from build123d import *

# Parameters (mm, degrees)
SKETCH1_W           = 12.7
SKETCH1_H           = 12.7
SKETCH1_R           = 1.905
BOSS_EXTRUDE1_DEPTH = 2.54
SKETCH2_W           = 1.791864934
SKETCH2_H           = 1.49598957
BOSS_EXTRUDE2_DEPTH = 10.16
SKETCH3_R           = 1.375
CUT_EXTRUDE1_DEPTH  = 17.896123524
FILLET1_R           = 1.016


with BuildPart() as part:
    # Sketch1 → Boss-Extrude1 (new body)
    with BuildSketch(Plane(origin=(0, 0, 0), x_dir=(1, 0, 0), z_dir=(0, 1, 0))):
        Rectangle(SKETCH1_W, SKETCH1_H)
        with Locations(Location((-3.175, 3.175, 0), (0, 0, 270))):
            Circle(SKETCH1_R, mode=Mode.SUBTRACT)
        with Locations(Location((3.175, 3.175, 0), (0, 0, 90))):
            Circle(SKETCH1_R, mode=Mode.SUBTRACT)
        with Locations(Location((3.175, -3.175, 0), (0, 0, 270))):
            Circle(SKETCH1_R, mode=Mode.SUBTRACT)
        with Locations(Location((-3.175, -3.175, 0), (0, 0, 90))):
            Circle(SKETCH1_R, mode=Mode.SUBTRACT)
    extrude(amount=BOSS_EXTRUDE1_DEPTH)

    # Sketch2 → Boss-Extrude2 (add)
    with BuildSketch(Plane(origin=(0, 2.54, 0), x_dir=(1, 0, 0), z_dir=(0, 1, 0))):
        Polygon((-1.016, 0.747994785), (-1.016, 2.249760645), (-2.807864934, 0.747994785), align=None)
        with Locations((-1.911932467, 0)):
            Rectangle(SKETCH2_W, SKETCH2_H)
        Polygon((-1.016, -2.249760645), (-1.016, -0.747994785), (-2.807864934, -0.747994785), align=None)
        Polygon((2.807864934, 0.747994785), (1.016, 2.249760645), (1.016, 0.747994785), align=None)
        with Locations((1.911932467, 0)):
            Rectangle(SKETCH2_W, SKETCH2_H)
        Polygon((2.807864934, -0.747994785), (1.016, -0.747994785), (1.016, -2.249760645), align=None)
    extrude(amount=BOSS_EXTRUDE2_DEPTH)

    # Sketch3 → Cut-Extrude1 (cut, through all)
    with BuildSketch(Plane(origin=(2.807864934, 0, 0), x_dir=(0, 0, -1), z_dir=(1, 0, 0))):
        with Locations(Location((0, 6.35, 0), (0, 0, 57.043905398))):
            Circle(SKETCH3_R)
    extrude(amount=-CUT_EXTRUDE1_DEPTH, mode=Mode.SUBTRACT)

    # Fillet1
    fillet1_edges = [part.edges().sort_by_distance(p)[0] for p in [
        (-6.35, 2.54, 0),
        (0, 2.54, 6.35),
        (6.35, 2.54, 0),
        (6.35, 1.27, 6.35),
        (-6.35, 1.27, 6.35),
        (-6.35, 1.27, -6.35),
        (6.35, 1.27, -6.35),
        (0, 2.54, -6.35),
    ]]
    fillet(fillet1_edges, radius=FILLET1_R)


solid = part.part
Read the model definition and answer for the solid it produces. Units are mm, in the model's axes. A direction names the side the tool comes from. Round coordinates to 2 decimals unless told otherwise and drop trailing zeros. Write each loop counter-clockwise with the first axis right and the second up, starting at its lowest first coordinate (ties: lowest second). Pieces come first, ordered by that corner, then holes.
Q1. Find section B-B on z = -0.5. Determine the outline of the cut face in (x, y), and give its area (3 significant figures).
Values:
outline: (-6.35, 0) - (6.35, 0) - (6.35, 1.52) arc R1.02 ccw to (5.33, 2.54) - (2.81, 2.54) - (2.81, 5.07) - (1.02, 5.07) - (1.02, 2.54) - (-1.02, 2.54) - (-1.02, 5.07) - (-2.81, 5.07) - (-2.81, 2.54) - (-5.33, 2.54) arc R1.02 ccw to (-6.35, 1.52) - close; (-2.81, 7.63) - (-1.02, 7.63) - (-1.02, 12.7) - (-2.81, 12.7) - close; (1.02, 7.63) - (2.81, 7.63) - (2.81, 12.7) - (1.02, 12.7) - close
area: 59.0 mm2
Q2. The mould has two halves that part along X. Classify faces 1 (the face through (6, 0.8, -6.1)), 2 (the face through (-3.905, 1.252, -1.415)), 3 (the face through (0, 0, 0)), 4 (the face through (5.064, 1.252, 2.927)): released by +X, released by -X, zero draft, split by the parting line, or undercut.
Values:
face 1: released by +X
face 2: undercut
face 3: zero draft
face 4: undercut
Q3. Straight lines are drawn through the part: line 1 (X direction, y = 2.75, z = 0); line 2 (Z direction, x = -2.5, y = 0.5); line 3 (Y direction, x = -1.25, z = -0.75). For each, find the intervals that lie inside material, in ascending order.
Values:
line 1: x = -2.81 to -1.02, 1.02 to 2.81
line 2: z = -6.35 to -4.96, -1.39 to 1.39, 4.96 to 6.35
line 3: y = 0 to 5.2, 7.5 to 12.7
Q4. Find section C-C on y = 7. Determine the outline of the cut face in (x, z), and give its area (3 significant figures).
Values:
outline: (-2.25, -1.21) - (-1.02, -2.25) - (-1.02, -1.21) - close; (-2.25, 1.21) - (-1.02, 1.21) - (-1.02, 2.25) - close; (1.02, -2.25) - (2.25, -1.21) - (1.02, -1.21) - close; (1.02, 1.21) - (2.25, 1.21) - (1.02, 2.25) - close
area: 2.57 mm2
Q5. Find section D-D on x = 3.5. Determine the outline of the cut face in (y, z), and give its area (3 significant figures).
Values:
outline: (0, -6.35) - (1.52, -6.35) arc R1.02 ccw to (2.54, -5.33) - (2.54, -5.05) - (0, -5.05) - close; (0, -1.3) - (2.54, -1.3) - (2.54, 1.3) - (0, 1.3) - close; (0, 5.05) - (2.54, 5.05) - (2.54, 5.33) arc R1.02 ccw to (1.52, 6.35) - (0, 6.35) - close
area: 12.7 mm2
Q6. Flat-ended cylindrical pins translate along their axes: P1, Ø1.2, axis at y = 3.5, z = 0, coming from the +X side; P2, Ø3, axis at x = 3, y = 8.5, coming from the +Z side; P3, Ø1.6, axis at y = 4.5, z = 0, coming from the -X side. Find the tip coordinate at first contact, or state that the pin passes through.
Values:
P1: stops at x = 2.81
P2: stops at z = 1.84
P3: stops at x = -2.81
Q7. A tool of negligible diameter and unlimited length cuts with its end or side. For faces 5 (the face through (-1.9, 7.55, -1.51)), 6 (the face through (-1.016, 9, 0)), 7 (the face through (1.9, 7.55, 1.51)), from which of +Z, -Z, +X, -X, +Y, -Y can it reach the whole face along a straight path? Write none if from no direction.
Values:
face 5: -Z, -X, +Y
face 6: +Z, -Z, +Y
face 7: +Z, +X, +Y
Q8. Find section A-A on y = 3.25. Determine the outline of the cut face in (x, z), and give its area (3 significant figures).
Values:
outline: (-2.81, -0.75) - (-1.02, -2.25) - (-1.02, 2.25) - (-2.81, 0.75) - close; (1.02, -2.25) - (2.81, -0.75) - (2.81, 0.75) - (1.02, 2.25) - close
area: 10.7 mm2
